Autodesk Inventor part; units mm, degrees
ref_plane "YZ Plane" through (0, 0, 0) normal (1, 0, 0) x (0, 1, 0)
ref_plane "XZ Plane" through (0, 0, 0) normal (0, 1, 0) x (-1, 0, 0)
ref_plane "XY Plane" through (0, 0, 0) normal (0, 0, 1) x (1, 0, 0)
ref_plane "Work Plane1" through (0, 0, 0) normal (0, 0, 1) x (1, 0, 0)
sketch "Sketch1" plane through (0, 0, 0) normal (0, 0, 1) x (1, 0, 0)
  circle A0 centre (25, -136.9573) radius 110
  line L0 (-96.6901, -226.845) -> (-113.6901, -197.4001)
  line L1 (-101.8073, -229.7994) -> (-118.8073, -200.3545)
  line L2 (163.6901, -197.4001) -> (146.6901, -226.845)
  line L3 (168.8073, -200.3545) -> (151.8073, -229.7994)
  line L4 (8, 13.3733) -> (42, 13.3733)
  line L5 (8, 19.2822) -> (42, 19.2822)
  line L6 (25, -136.9573) -> (25, 19.2822)
  line L7 (25, -136.9573) -> (160.3073, -215.077)
  line L8 (25, -136.9573) -> (-110.3073, -215.077)
  line L9 (-10, -135.9724) -> (-10, 19.2822)
  line L10 (60, -135.9724) -> (60, 19.2822)
  line L11 (43.3529, -107.1388) -> (177.8073, -184.7661)
  line L12 (8.3529, -167.7605) -> (142.8073, -245.3879)
  line L13 (41.6471, -167.7605) -> (-92.8073, -245.3879)
  line L14 (6.6471, -107.1388) -> (-127.8073, -184.7661)
  arc A1 (142.8073, -245.3879) -> (177.8073, -184.7661) centre (160.3073, -215.077) ccw
  arc A2 (60, 19.2822) -> (-10, 19.2822) centre (25, 19.2822) ccw
  arc A3 (-127.8073, -184.7661) -> (-92.8073, -245.3879) centre (-110.3073, -215.077) ccw
  line L15 (25, -177.3718) -> (76.9615, -207.3718)
  line L16 (-10, -116.75) -> (-61.9615, -146.75)
  line L17 (-10, -116.75) -> (-10, -56.75)
  line L18 (60, -116.75) -> (60, -56.75)
  line L19 (60, -116.75) -> (111.9615, -146.75)
  line L20 (111.9615, -146.75) -> (60, -56.75)
  line L21 (-10, -56.75) -> (-61.9615, -146.75)
  line L22 (25, -177.3718) -> (-26.9615, -207.3718)
  line L23 (-26.9615, -207.3718) -> (76.9615, -207.3718)
  circle A4 centre (25, -136.9573) radius 40.4145
  point P0 (0, 0)
extrude "Extrusion1" add sketch "Sketch1" along normal blind 3 contours L10 A4 L6 A0 | A0 L9 A2 L10 | L11 A1 L12 A0 | A0 L7 A4 L11 | L6 A4 L9 A0 | L20 L11 L10 | A0 L12 A4 L7 | L14 A4 L8 A0 | A0 L13 A3 L14 | L9 L14 L21 | A0 L8 A4 L13 | L23 L13 L12
sketch "Sketch3" plane through (0, 0, 0) normal (0, 0, -1) x (-1, 0, 0)
  circle A0 centre (-40, -1.2646) radius 1.5
  circle A1 centre (-10, -1.2646) radius 1.5
  circle A2 centre (-10, 31.4848) radius 1.5
  circle A3 centre (-40, 31.4848) radius 1.5
  circle A4 centre (113.3751, -234.1687) radius 1.5
  circle A5 centre (85.0133, -217.794) radius 1.5
  circle A6 centre (100.0133, -191.8132) radius 1.5
  circle A7 centre (128.3751, -208.1879) radius 1.5
  circle A8 centre (-135.0133, -217.794) radius 1.5
  circle A9 centre (-163.3751, -234.1687) radius 1.5
  circle A10 centre (-178.3751, -208.1879) radius 1.5
  circle A11 centre (-150.0133, -191.8132) radius 1.5
  point P0 (0, 0)
extrude "Extrusion2" cut sketch "Sketch3" against normal blind 6
properties part number "Bund"
Verification items for the finished model (mm, model axes). A direction names the side the tool comes from. Give positions to 0.01 mm unless a question says otherwise; leave off trailing zeros. Write each loop counter-clockwise with the first axis right and the second up, starting at its lowest first coordinate (ties: lowest second). Pieces come first, ordered by that corner, then holes. Notation, with made-up numbers: M 38.25,73 L 87.25,73 A37 cw 87.25,112 Z; hole C 52.5,-13.75 d10. An arc over 180 degrees is marked long. One line per question, with ' | ' between items.
1) Section check B-B on y = -127.5. Enter the section's corners in (x, z).
Result:
outline: M -50.85,0 L -14.29,0 L -14.29,3 L -50.85,3 Z; M 64.29,0 L 100.85,0 L 100.85,3 L 64.29,3 Z
2) Thickness scan on line 1 along X through (y, z) = (-234.5, 1.65); line 2 along Y through (x, z) = (10, 1.5); line 3 along X through (y, z) = (-219, 1.8). Record the ranges inside material, lowest first. Write a range as [from, to].
Result:
line 1: x = [-139.42, -114.84], [-111.91, -73.95], [123.95, 161.91], [164.84, 189.42] | line 2: y = [-207.37, -174.49], [-99.43, -2.76], [0.24, 29.98], [32.98, 50.9] | line 3: x = [-145.09, -85.91], [-84.12, -47.1], [97.1, 134.12], [135.91, 195.09]
3) Section check C-C on z = 1.2. State how many separate pieces and enclosed holes the cut face has, plus the area to 3 significant figures.
Result:
separate pieces: 1 | enclosed holes: 13 | area: 35,900 mm2
4) Set-up check for faces 1 (the cylindrical face through (46.727, -171.035, 1.479)), 2 (the flat face through (109.4, -226.1, 1.5)): record each of +Z, -Z, +X, -X, +Y, -Y from which the full face is reachable in a straight line by a thin tool's end or side.
Result:
face 1: +Z, -Z | face 2: +Z, -Z, -Y
5) Gauge pin test, flat ends, axial feed: pin 1 Ø1.5 at (y, z) = (-78.5, 2.5) entering from +X; pin 2 Ø1.5 at (y, z) = (-155.5, 1) entering from -X; pin 3 Ø0.9 at (x, z) = (23.5, 1.5) entering from -Y. Record the tip position at first contact, or that the pin passes through.
Result:
pin 1: stops at x = 72.99 | pin 2: stops at x = -78.42 | pin 3: stops at y = -207.37
6) Section check D-D on y = 15.5. Enter the section's corners in (x, z), plus the area to 3 significant figures.
Result:
outline: M -10,0 L 60,0 L 60,3 L -10,3 Z | area: 210 mm2
7) Mould release check, pull along X, two halves, no side actions. Record for faces 3 (the flat face through (-14, -154, 3)), 4 (the flat face through (86.344, -102.38, 1.479)), 5 (the flat face through (-59.4, -226.1, 1.5)): released by +X, released by -X, zero draft, split by the parting line, or undercut.
Result:
face 3: zero draft | face 4: released by +X | face 5: undercut
8) Section check A-A on x = 25. Enter the section's corners in (y, z), plus the area to 3 significant figures.
Result:
outline: M -207.37,0 L -177.37,0 L -177.37,3 L -207.37,3 Z; M -96.54,0 L 54.28,0 L 54.28,3 L -96.54,3 Z | area: 542 mm2
